CAD build for the part. Positions are in the model's coordinates, mm. Coordinates: 2 decimals unless noted, no trailing zeros. Order: outer loops, then holes, each group sorted by start corner. A loop starts at its lowest first (then second) coordinate and runs counter-clockwise, first axis right, second up. Notation, with made-up numbers: M 85,14.25 L 97,14.25 A15 ccw 97,25.25 Z; hole C -10,-2.5 d10. An arc over 180 degrees is marked long. One line per item, written item: value.
Autodesk Inventor part; units mm, degrees
ref_plane "Work Plane1" through (-358.775, 358.775, 0) normal (0.7071, 0.7071, 0) x (0, 0, 1)
ref_plane "YZ Plane" through (0, 0, 0) normal (1, 0, 0) x (0, 1, 0)
ref_plane "XZ Plane" through (0, 0, 0) normal (0, 1, 0) x (-1, 0, 0)
sketch "Sketch1" plane through (0, 0, 0) normal (0, 0, 1) x (1, 0, 0)
  line L0 (-358.775, -358.775) -> (358.775, -358.775)
  line L1 (358.775, -358.775) -> (358.775, 358.775)
  line L2 (358.775, 358.775) -> (-358.775, 358.775)
  line L3 (-358.775, 358.775) -> (-358.775, -358.775)
  line L4 (-358.775, -358.775) -> (358.775, 358.775) construction
  line L5 (358.775, -358.775) -> (-358.775, 358.775) construction
  point P0 (0, 0)
  dimension "d0" = 717.55
  dimension "d1" = 717.55
extrude "Extrusion1" add sketch "Sketch1" along normal blind 12.7
sketch "Sketch2" plane through (0, 0, 12.7) normal (0, 0, 1) x (1, 0, 0)
  circle A0 centre (-293.5432, -293.5432) radius 6.35
  line L0 (-358.775, 358.775) -> (-358.775, -358.775)
  line L1 (-293.5432, -293.5432) -> (293.5432, -293.5432)
  line L2 (293.5432, -293.5432) -> (293.5432, 293.5432)
  line L3 (293.5432, 293.5432) -> (-293.5432, 293.5432)
  line L4 (-293.5432, 293.5432) -> (-293.5432, -293.5432)
  line L5 (-293.5432, -293.5432) -> (293.5432, 293.5432) construction
  line L6 (293.5432, -293.5432) -> (-293.5432, 293.5432) construction
  point P0 (0, 0)
  dimension "d4" = 12.7
  dimension "d6" = 587.0864
extrude "Extrusion2" add sketch "Sketch2" along normal blind 12.7 contours L1 L4 A0 | A0 L4 L1
pattern_linear "Rectangular Pattern1" count 10 spacing 65.2318 along (1, 0, 0) of "Extrusion2"
pattern_linear "Rectangular Pattern2" count 10 spacing 65.2318 along (0, 1, 0) of "Extrusion2"
ref_plane "Work Plane1" through (-358.775, 358.775, 0) normal (0.7071, 0.7071, 0) x (0, 0, 1)
mirror "Mirror1" about plane through (-358.775, 358.775, 0) normal (0.7071, 0.7071, 0) of "Extrusion2", "Rectangular Pattern1", "Rectangular Pattern2"
properties part number "connection_plate"
Q1. Drill centre lines: line 1 along X through (y, z) = (-167.5, 24.25); line 2 along X through (y, z) = (-96, 20); line 3 along Z through (x, y) = (-110.5, 278). Where is each one in solid material? Low to high.
Recorded:
line 1: x = -298.1 to -288.98, 288.98 to 298.1
line 2: x = -299.62 to -287.47, 287.47 to 299.62
line 3: z = 0 to 12.7
Q2. Mould opens along X. For faces 1 (the face through (-5, 5, 12.7)), 2 (the face through (-5, 5, 0)) say: released by +X, released by -X, zero draft, split by the parting line, or undercut.
Recorded:
face 1: undercut
face 2: zero draft
Q3. Slice it at A-A (x = -312). List the corners of the cut face in (y, z) (3 decimals).
Recorded:
outline: M -358.775,0 L 358.775,0 L 358.775,12.7 L -358.775,12.7 Z
Q4. Pin check, flat tip, straight feed: pin 1 Ø3 at (x, z) = (-100.5, 19) entering from +Y. Stop position of the tip, or through.
Recorded:
pin 1: stops at y = 299.79
